The listing builds one solid part. Answer for the finished solid, in the listing's coordinates (mm). Coordinates: 2 decimals unless noted, no trailing zeros. Order: outer loops, then holes, each group sorted by start corner. A loop starts at its lowest first (then second) coordinate and runs counter-clockwise, first axis right, second up. Notation, with made-up numbers: (7.5, 33) -> (15.5, 33) arc R22 cw to (15.5, 67) -> close; hole circle Ø3 at (-23, -15). An arc over 180 degrees is marked (long way). Return JSON: item names as keys, results as strings.
from build123d import *

# Parameters (mm, degrees)
F1_DEPTH = 15.75
F2_R     = 2.5
F3_DEPTH = 15.751


with BuildPart() as f1:
    # F0 (on Top) → F1 (new body)
    with BuildSketch(Plane.XY):
        with BuildLine():
            ThreePointArc((18, 20.15), (0, 38.15), (-18, 20.15))
            Line((-18, 20.15), (-18, -20.15))
            ThreePointArc((-18, -20.15), (0, -38.15), (18, -20.15))
            Line((18, -20.15), (18, 20.15))
        make_face()
    extrude(amount=F1_DEPTH)

    # F2 (on face) → F3 (cut, through all)
    with BuildSketch(Plane.XY.offset(15.75)):
        with Locations((0, 29.15)):
            Circle(F2_R)
        with Locations((0, -29.15)):
            Circle(F2_R)
    extrude(amount=-F3_DEPTH, mode=Mode.SUBTRACT)


solid = f1.part
1. Each of these flat-tipped pins is pushed along its axis until it touches: pin 1 Ø6 at (x, z) = (-10.5, 2) entering from +Y; pin 2 Ø1.5 at (x, z) = (10.5, 4.5) entering from +Y; pin 3 Ø1 at (x, z) = (-5.5, 11.5) entering from +Y. Where does it stop, or does it pass through?
Answer block:
{"pin 1": "stops at y = 36.51", "pin 2": "stops at y = 35.28", "pin 3": "stops at y = 37.44"}
2. The part is cut by section A-A on x = 0. Give the vertices of the cut face in (y, z), and give its area (3 significant figures).
Answer block:
{"outline": "(-38.15, 0) -> (-31.65, 0) -> (-31.65, 15.75) -> (-38.15, 15.75) -> close; (-26.65, 0) -> (26.65, 0) -> (26.65, 15.75) -> (-26.65, 15.75) -> close; (31.65, 0) -> (38.15, 0) -> (38.15, 15.75) -> (31.65, 15.75) -> close", "area": "1,040 mm2"}
3. Consider line 1 (Y direction, x = 0, z = 11); line 2 (Y direction, x = -2, z = 8); line 3 (Y direction, x = -14, z = 10). Determine where each line is inside the solid, lowest interval first. Write a range as from..to.
Answer block:
{"line 1": "y = -38.15..-31.65, -26.65..26.65, 31.65..38.15", "line 2": "y = -38.04..-30.65, -27.65..27.65, 30.65..38.04", "line 3": "y = -31.46..31.46"}
4. The part is cut by section C-C on z = 14.5. Give the vertices of the cut face in (x, y).
Answer block:
{"outline": "(-18, -20.15) arc R18 ccw to (18, -20.15) -> (18, 20.15) arc R18 ccw to (-18, 20.15) -> close; hole circle Ø5 at (0, -29.15); hole circle Ø5 at (0, 29.15)"}
5. Determine the mould class of faces 1 (the face through (-0.5, -31.6, 8)), 2 (the face through (-18, 0, 8)), 3 (the face through (-0.396, -38.146, 7.765)) for opening direction X: pulls with the +X half, pulls with the -X half, needs draft (parallel to the pull), parting line crosses it, or undercut.
Answer block:
{"face 1": "undercut", "face 2": "pulls with the -X half", "face 3": "parting line crosses it"}
6. The part is cut by section B-B on y = -29.15. Give the vertices of the cut face in (x, z), and give its area (3 significant figures).
Answer block:
{"outline": "(-15.59, 0) -> (-2.5, 0) -> (-2.5, 15.75) -> (-15.59, 15.75) -> close; (2.5, 0) -> (15.59, 0) -> (15.59, 15.75) -> (2.5, 15.75) -> close", "area": "412 mm2"}
